```python
from build123d import *

# Parameters (mm, degrees)
SKETCH_1_W                    = 5
SKETCH_1_H                    = 10
EXTRUDE_297_DEPTH             = 2.5
SKETCH_2_W                    = 2.5
SKETCH_2_H                    = 8
EXTRUDE_2_DEPTH               = 8
HOLE_WIZARD_M2_5_2_D          = 2.7
EXTRUDE_1_DEPTH               = 3.8
FILLET_1_RADIUS               = 4
FILLET_1_LENGTH               = 2.5
FILLET_1_OF_MIRROR_1_2_RADIUS = 4
FILLET_1_OF_MIRROR_1_2_LENGTH = 2.5
SKETCH_13_W                   = 5
SKETCH_13_H                   = 2.5
EXTRUDE_3_DEPTH               = 5
SKETCH_15_W                   = 2.8
SKETCH_15_H                   = 14
CUT_EXTRUDE_2383_DEPTH        = 0.9
FILLET_2_R                    = 0.5
SKETCH_16_W                   = 5
SKETCH_16_H                   = 1
EXTRUDE_4_DEPTH               = 0.35
SKETCH_17_W                   = 5
SKETCH_17_H                   = 1.5
EXTRUDE_5_DEPTH               = 5
CUT_EXTRUDE_1_REACH           = 21.02
SKETCH_18_R                   = 1.25
FILLET_3_RADIUS               = 2.5
FILLET_3_LENGTH               = 1.5
FILLET_4_R                    = 0.4
FILLET_5_R                    = 1
CUT_EXTRUDE_2_REACH           = 21.09
SKETCH_19_W                   = 2.8
SKETCH_19_H                   = 2


with BuildPart() as part:
    # 草图1 → Extrude 297 (new body)
    with BuildSketch(Plane.XY):
        Rectangle(SKETCH_1_W, SKETCH_1_H)
    extrude(amount=EXTRUDE_297_DEPTH)

    # 草图2 → 凸台-拉伸2 (add)
    with BuildSketch(Plane(origin=(2.5, 0, 0), x_dir=(0, 0, -1), z_dir=(1, 0, 0))):
        with Locations((-1.25, 0)):
            Rectangle(SKETCH_2_W, SKETCH_2_H)
    extrude_2 = extrude(amount=EXTRUDE_2_DEPTH)

    # M2.5 间隙孔2 (through all)
    with Locations(Plane.XY.offset(2.5)):
        with Locations((6.5, 0)):
            hole_wizard_m2_5_2 = Hole(HOLE_WIZARD_M2_5_2_D / 2)

    # 草图11 → 拉伸-薄壁1 (add)
    with BuildSketch(Plane(origin=(0, 0, 0), x_dir=(-1, 0, 0), z_dir=(0, 0, -1))):
        Polygon((-4.508141571, 3.45), (-8.491858429, 3.45), (-10.483716857, 0), (-8.491858429, -3.45), (-4.508141571, -3.45), (-2.516283143, 0), align=None)
        Polygon((-4.970021787, 2.65), (-8.029978213, 2.65), (-9.559956427, 0), (-8.029978213, -2.65), (-4.970021787, -2.65), (-3.440043573, 0), align=None, mode=Mode.SUBTRACT)
    extrude_1 = extrude(amount=EXTRUDE_1_DEPTH)

    # 圆角1: full round fillet: the end face becomes a half cylinder, R = half its width
    fillet_1_face = Plane((10.5, 0, 1.25), x_dir=(0, 0, 1), z_dir=(1, 0, 0))  # on the end face: x along it, z out of the body
    fillet_1_slab = fillet_1_face.offset(-FILLET_1_RADIUS / 2) * Box(FILLET_1_LENGTH, 2 * FILLET_1_RADIUS, FILLET_1_RADIUS, mode=Mode.PRIVATE)  # the body's end, R deep
    fillet_1_round = Plane((6.5, 0, 1.25), x_dir=(1, 0, 0), z_dir=(0, 0, 1)) * Cylinder(FILLET_1_RADIUS, FILLET_1_LENGTH, mode=Mode.PRIVATE)  # its axis R under the face
    add(fillet_1_slab - fillet_1_round, mode=Mode.SUBTRACT)

    # 镜向1: 凸台-拉伸2, M2.5 间隙孔2, 拉伸-薄壁1 across plane
    add(extrude_2.mirror(Plane(origin=(0, 0, 0), x_dir=(0, 0, 1), z_dir=(1, 0, 0))))
    add(hole_wizard_m2_5_2.mirror(Plane(origin=(0, 0, 0), x_dir=(0, 0, 1), z_dir=(1, 0, 0))), mode=Mode.SUBTRACT)
    add(extrude_1.mirror(Plane(origin=(0, 0, 0), x_dir=(0, 0, 1), z_dir=(1, 0, 0))))

    # 圆角1 of Mirror 1 2: full round fillet: the end face becomes a half cylinder, R = half its width
    fillet_1_of_mirror_1_2_face = Plane((-10.5, 0, 1.25), x_dir=(0, 0, 1), z_dir=(-1, 0, 0))  # on the end face: x along it, z out of the body
    fillet_1_of_mirror_1_2_slab = fillet_1_of_mirror_1_2_face.offset(-FILLET_1_OF_MIRROR_1_2_RADIUS / 2) * Box(FILLET_1_OF_MIRROR_1_2_LENGTH, 2 * FILLET_1_OF_MIRROR_1_2_RADIUS, FILLET_1_OF_MIRROR_1_2_RADIUS, mode=Mode.PRIVATE)  # the body's end, R deep
    fillet_1_of_mirror_1_2_round = Plane((-6.5, 0, 1.25), x_dir=(-1, 0, 0), z_dir=(0, 0, 1)) * Cylinder(FILLET_1_OF_MIRROR_1_2_RADIUS, FILLET_1_OF_MIRROR_1_2_LENGTH, mode=Mode.PRIVATE)  # its axis R under the face
    add(fillet_1_of_mirror_1_2_slab - fillet_1_of_mirror_1_2_round, mode=Mode.SUBTRACT)

    # 草图13 → 凸台-拉伸3 (add)
    with BuildSketch(Plane.XZ.offset(5)):
        with Locations((0, 1.25)):
            Rectangle(SKETCH_13_W, SKETCH_13_H)
    extrude(amount=EXTRUDE_3_DEPTH)

    # 草图15 → Cut-Extrude 2383 (cut)
    with BuildSketch(Plane.XY.offset(2.5)):
        with Locations((0, -2)):
            Rectangle(SKETCH_15_W, SKETCH_15_H)
    extrude(amount=-CUT_EXTRUDE_2383_DEPTH, mode=Mode.SUBTRACT)

    # 圆角2
    fillet_2_edges = [part.edges().sort_by_distance(p)[0] for p in [
        (0, 5, 1.6),
    ]]
    fillet(fillet_2_edges, radius=FILLET_2_R)

    # 草图16 → 凸台-拉伸4 (add)
    with BuildSketch(Plane.XY.offset(2.5)):
        with Locations((0, -9.5)):
            Rectangle(SKETCH_16_W, SKETCH_16_H)
    extrude(amount=EXTRUDE_4_DEPTH)

    # 草图17 → 凸台-拉伸5 (add)
    with BuildSketch(Plane.XZ.offset(10)):
        with Locations((0, 2.1)):
            Rectangle(SKETCH_17_W, SKETCH_17_H)
    extrude(amount=EXTRUDE_5_DEPTH)

    # 草图18 → 切除-拉伸1 (cut, up to next)
    with BuildSketch(Plane(origin=(0, 0, 1.35), x_dir=(-1, 0, 0), z_dir=(0, 0, -1)), mode=Mode.PRIVATE) as cut_extrude_1_sk1:
        with Locations((0, -12.5)):
            Circle(SKETCH_18_R)
    cut_extrude_1_tool1 = extrude(cut_extrude_1_sk1.sketch, amount=-CUT_EXTRUDE_1_REACH, mode=Mode.PRIVATE) & part.part
    add(cut_extrude_1_tool1.solids().sort_by_distance((0, -12.5, 1.35))[0], mode=Mode.SUBTRACT)

    # 圆角3: full round fillet: the end face becomes a half cylinder, R = half its width
    fillet_3_face = Plane((0, -15, 2.1), x_dir=(0, 0, -1), z_dir=(0, -1, 0))  # on the end face: x along it, z out of the body
    fillet_3_slab = fillet_3_face.offset(-FILLET_3_RADIUS / 2) * Box(FILLET_3_LENGTH, 2 * FILLET_3_RADIUS, FILLET_3_RADIUS, mode=Mode.PRIVATE)  # the body's end, R deep
    fillet_3_round = Plane((0, -12.5, 2.1), x_dir=(0, -1, 0), z_dir=(0, 0, -1)) * Cylinder(FILLET_3_RADIUS, FILLET_3_LENGTH, mode=Mode.PRIVATE)  # its axis R under the face
    add(fillet_3_slab - fillet_3_round, mode=Mode.SUBTRACT)

    # 圆角4
    fillet_4_edges = [part.edges().sort_by_distance(p)[0] for p in [
        (1.25, -12.5, 2.85),
        (1.25, -12.5, 1.35),
        (0, -9, 2.85),
    ]]
    fillet(fillet_4_edges, radius=FILLET_4_R)

    # 圆角5
    fillet_5_edges = [part.edges().sort_by_distance(p)[0] for p in [
        (0, -10, 0),
    ]]
    fillet(fillet_5_edges, radius=FILLET_5_R)

    # 草图19 → 切除-拉伸2 (cut, up to next)
    with BuildSketch(Plane.XY.offset(1.6), mode=Mode.PRIVATE) as cut_extrude_2_sk1:
        with Locations((0, -8)):
            Rectangle(SKETCH_19_W, SKETCH_19_H)
    cut_extrude_2_tool1 = extrude(cut_extrude_2_sk1.sketch, amount=-CUT_EXTRUDE_2_REACH, mode=Mode.PRIVATE) & part.part
    add(cut_extrude_2_tool1.solids().sort_by_distance((0, -8, 1.6))[0], mode=Mode.SUBTRACT)


solid = part.part
```
Check sheet for the modelled part. Datum: model origin and axes. Units: mm. A direction names the side the tool comes from. Round coordinates to 2 decimals unless told otherwise and drop trailing zeros. Order: outer loops, then holes, each group sorted by start corner. A loop starts at its lowest first (then second) coordinate and runs counter-clockwise, first axis right, second up. Notation, with made-up numbers: (24, -2.75) -> (78, -2.75) arc R23 ccw to (78, 25.25) -> close; hole circle Ø4 at (42.5, 70.5). An arc over 180 degrees is marked (long way). One line per item, written item: value. Start each with the question number.
Q1. Thickness scan on line 1 (Y direction, x = 6.5, z = 1.5); line 2 (X direction, y = -4.5, z = 1.75); line 3 (X direction, y = -2.25, z = -0.5). Record the ranges inside material, lowest first.
Q2. Mould release check, pull along Y, two halves, no side actions. Record for faces 4 (the face through (7, -3.45, -2)), 5 (the face through (5, 0, 2.5)), 6 (the face through (6, 2.65, -2)): pulls with the +Y half, pulls with the -Y half, needs draft (parallel to the pull), parting line crosses it, or undercut.
Q3. Cross-section at D-D (z = 2). Record the boundary of the cut face in (x, y).
Q4. Cross-section at C-C (x = 0). Record the boundary of the cut face in (y, z), and give its area (3 significant figures).
Q5. Cross-section at B-B (y = -8). Record the boundary of the cut face in (x, z), and give its area (3 significant figures).
Q6. Set-up check for faces 1 (the face through (8, 1, 0)), 2 (the face through (4, 4, 1)), 3 (the face through (0, -9, 1)): record each of +Z, -Z, +X, -X, +Y, -Y from which the full face is reachable in a straight line by a thin tool's end or side.
Q7. Cross-section at A-A (z = -2.25). Record the boundary of the cut face in (x, y), and give its area (3 significant figures).
Q8. Gauge pin test, flat ends, axial feed: pin 1 Ø2.5 at (x, y) = (6.5, 0) entering from -Z; pin 2 Ø2 at (x, y) = (0.5, -2.5) entering from +Z; pin 3 Ø2.5 at (x, z) = (-7, -2) entering from -Y; pin 4 Ø3 at (x, y) = (-3.5, -6.5) entering from -Z. Record the tip position at first contact, or that the pin passes through.
Completed:
1. line 1: y = -4 to -1.35, 1.35 to 4
1. line 2: x = -2.5 to -1.4, 1.4 to 2.5
1. line 3: x = -9.18 to -8.26, -4.74 to -3.82, 3.82 to 4.74, 8.26 to 9.18
2. face 4: pulls with the -Y half
2. face 5: needs draft
2. face 6: undercut
3. outline: (-6.5, -4) -> (-2.5, -4) -> (-2.5, -12.5) arc R2.5 ccw to (2.5, -12.5) -> (2.5, -4) -> (6.5, -4) arc R4 ccw to (6.5, 4) -> (2.5, 4) -> (2.5, 5) -> (1.4, 5) -> (1.4, -9) -> (-1.4, -9) -> (-1.4, 5) -> (-2.5, 5) -> (-2.5, 4) -> (-6.5, 4) arc R4 ccw to start; hole circle Ø2.7 at (-6.5, 0); hole circle Ø2.5 at (0, -12.5); hole circle Ø2.7 at (6.5, 0)
4. outline: (-15, 1.35) -> (-14.15, 1.35) arc R0.4 ccw to (-13.75, 1.75) -> (-13.75, 2.45) arc R0.4 ccw to (-14.15, 2.85) -> (-15, 2.85) -> close; (-11.25, 1.75) arc R0.4 ccw to (-10.85, 1.35) -> (-10, 1.35) -> (-10, 1) arc R1 ccw to (-9, 0) -> (-9, 2.45) arc R0.4 ccw to (-9.4, 2.85) -> (-10.85, 2.85) arc R0.4 ccw to (-11.25, 2.45) -> close; (-7, 0) -> (5, 0) -> (5, 1.1) arc R0.5 ccw to (4.5, 1.6) -> (-7, 1.6) -> close
4. area: 25.4 mm²
5. outline: (-2.5, 0) -> (-1.4, 0) -> (-1.4, 2.5) -> (-2.5, 2.5) -> close; (1.4, 0) -> (2.5, 0) -> (2.5, 2.5) -> (1.4, 2.5) -> close
5. area: 5.50 mm²
6. face 1: -Z
6. face 2: +Z, -Z, +X, +Y
6. face 3: +Z, -Z
7. outline: (-10.48, 0) -> (-8.49, -3.45) -> (-4.51, -3.45) -> (-2.52, 0) -> (-4.51, 3.45) -> (-8.49, 3.45) -> close; (2.52, 0) -> (4.51, -3.45) -> (8.49, -3.45) -> (10.48, 0) -> (8.49, 3.45) -> (4.51, 3.45) -> close; hole (-9.56, 0) -> (-8.03, -2.65) -> (-4.97, -2.65) -> (-3.44, 0) -> (-4.97, 2.65) -> (-8.03, 2.65) -> close; hole (3.44, 0) -> (4.97, -2.65) -> (8.03, -2.65) -> (9.56, 0) -> (8.03, 2.65) -> (4.97, 2.65) -> close
7. area: 33.8 mm²
8. pin 1: passes through
8. pin 2: stops at z = 2.5
8. pin 3: stops at y = -3.45
8. pin 4: stops at z = 0
